from build123d import *

# Parameters (mm, degrees)
SKETCH4_W           = 70
SKETCH4_H           = 80
SKETCH4_R           = 2.5
BOSS_EXTRUDE2_DEPTH = 4
SKETCH5_R           = 11.5
SKETCH5_R_2         = 1.5
SKETCH5_R_3         = 2.5
CUT_EXTRUDE2_DEPTH  = 5
FILLET1_R           = 5


with BuildPart() as part:
    # Sketch4 → Boss-Extrude2 (new body)
    with BuildSketch(Plane.XY):
        Rectangle(SKETCH4_W, SKETCH4_H)
        with Locations((-27, 7)):
            Circle(SKETCH4_R, mode=Mode.SUBTRACT)
        with Locations((27, 7)):
            Circle(SKETCH4_R, mode=Mode.SUBTRACT)
        with BuildLine():
            Line((-24.5, -34), (-24.5, -35))
            ThreePointArc((-24.5, -35), (-27, -37.5), (-29.5, -35))
            Line((-29.5, -35), (-29.5, -34))
            ThreePointArc((-29.5, -34), (-27, -31.5), (-24.5, -34))
        make_face(mode=Mode.SUBTRACT)
        with BuildLine():
            Line((24.5, -34), (24.5, -35))
            ThreePointArc((24.5, -35), (27, -37.5), (29.5, -35))
            Line((29.5, -35), (29.5, -34))
            ThreePointArc((29.5, -34), (27, -31.5), (24.5, -34))
        make_face(mode=Mode.SUBTRACT)
    extrude(amount=BOSS_EXTRUDE2_DEPTH)

    # Sketch5 → Cut-Extrude2 (cut, through all)
    with BuildSketch(Plane.XY.offset(4)):
        with Locations((0, 20.076696831)):
            Circle(SKETCH5_R)
        with Locations((-15.5, 35.576696831)):
            Circle(SKETCH5_R_2)
        with Locations((15.5, 35.576696831)):
            Circle(SKETCH5_R_2)
        with Locations((15.5, 4.576696831)):
            Circle(SKETCH5_R_2)
        with Locations((-15.5, 4.576696831)):
            Circle(SKETCH5_R_2)
        with Locations((0, -14.75)):
            Circle(SKETCH5_R_3)
        with BuildLine():
            Line((-8, -31.570071963), (8, -31.570071963))
            ThreePointArc((8, -31.570071963), (10.5, -34.070071963), (8, -36.570071963))
            Line((8, -36.570071963), (-8, -36.570071963))
            ThreePointArc((-8, -36.570071963), (-10.5, -34.070071963), (-8, -31.570071963))
        make_face()
        with BuildLine():
            Line((-13, -6.75), (-13, -22.75))
            ThreePointArc((-13, -22.75), (-15.5, -25.25), (-18, -22.75))
            Line((-18, -22.75), (-18, -6.75))
            ThreePointArc((-18, -6.75), (-15.5, -4.25), (-13, -6.75))
        make_face()
        with BuildLine():
            Line((13, -6.75), (13, -22.75))
            ThreePointArc((13, -22.75), (15.5, -25.25), (18, -22.75))
            Line((18, -22.75), (18, -6.75))
            ThreePointArc((18, -6.75), (15.5, -4.25), (13, -6.75))
        make_face()
    extrude(amount=-CUT_EXTRUDE2_DEPTH, mode=Mode.SUBTRACT)

    # Fillet1
    fillet1_edges = [part.edges().sort_by_distance(p)[0] for p in [
        (35, -40, 2),
        (-35, -40, 2),
        (-35, 40, 2),
        (35, 40, 2),
    ]]
    fillet(fillet1_edges, radius=FILLET1_R)


solid = part.part
Model file for the job. Use its own axes, mm. A direction names the side the tool comes from. Give positions to 0.01 mm unless a question says otherwise; leave off trailing zeros. Order: outer loops, then holes, each group sorted by start corner. A loop starts at its lowest first (then second) coordinate and runs counter-clockwise, first axis right, second up. Notation, with made-up numbers: M -5,-12.75 L 1,-12.75 A18 cw 1,9.25 Z; hole C 59,55.5 d9. An arc over 180 degrees is marked long. Put each result on its own line as item: value. Start each with the question number.
(1) Band-saw the part on B-B on y = -20. Give the cut face in (x, z).
(2) Drill centre lines: L1, parallel to Y at x = -15.5, z = 2.5; L2, parallel to Y at x = 0, z = 1.1; L3, parallel to X at y = -13, z = 2.75. Where is each one in solid material? Low to high. Write a range as [from, to].
(3) Band-saw the part on C-C on x = 15.5. Give the cut face in (y, z), then the cut area to 3 significant figures.
(4) Band-saw the part on A-A on x = 27. Give the cut face in (y, z), then the cut area to 3 significant figures.
(5) Band-saw the part on D-D on y = 22. Give the cut face in (x, z).
(6) Pull direction Y, two halves, no side cores. Call faces 1 (the face through (35, 0, 2)), 2 (the face through (0, 40, 2)), 3 (the face through (-18, -15, 2)): released by +Y, released by -Y, zero draft, split by the parting line, or undercut.
(7) Tool access for faces 4 (the face through (18, -15, 2)), 5 (the face through (33, -39, 2)): list every direction of +Z, -Z, +X, -X, +Y, -Y with a clear straight run to the whole face (end or side of a thin tool).
(8) Pin check, flat tip, straight feed: pin 1 Ø4.5 at (x, y) = (0, -14.75) entering from -Z. Stop position of the tip, or through.
Results below:
1. outline: M -35,0 L -18,0 L -18,4 L -35,4 Z; M -13,0 L 13,0 L 13,4 L -13,4 Z; M 18,0 L 35,0 L 35,4 L 18,4 Z
2. L1: y = [-40, -25.25], [-4.25, 3.08], [6.08, 34.08], [37.08, 40]
2. L2: y = [-40, -36.57], [-31.57, -17.25], [-12.25, 8.58], [31.58, 40]
2. L3: x = [-35, -18], [-13, -1.79], [1.79, 13], [18, 35]
3. outline: M -40,0 L -25.25,0 L -25.25,4 L -40,4 Z; M -4.25,0 L 3.08,0 L 3.08,4 L -4.25,4 Z; M 6.08,0 L 34.08,0 L 34.08,4 L 6.08,4 Z; M 37.08,0 L 40,0 L 40,4 L 37.08,4 Z
3. area: 212 mm2
4. outline: M -40,0 L -37.5,0 L -37.5,4 L -40,4 Z; M -31.5,0 L 4.5,0 L 4.5,4 L -31.5,4 Z; M 9.5,0 L 40,0 L 40,4 L 9.5,4 Z
4. area: 276 mm2
5. outline: M -35,0 L -11.34,0 L -11.34,4 L -35,4 Z; M 11.34,0 L 35,0 L 35,4 L 11.34,4 Z
6. face 1: zero draft
6. face 2: released by +Y
6. face 3: undercut
7. face 4: +Z, -Z
7. face 5: +Z, -Z, +X, -Y
8. pin 1: passes through
